Drawing for the job (mm, zero at the part's lowest x, y, z). A direction names the side the tool comes from. Round coordinates to 2 decimals unless told otherwise and drop trailing zeros. Write each loop counter-clockwise with the first axis right and the second up, starting at its lowest first coordinate (ties: lowest second). Pieces come first, ordered by that corner, then holes. Notation, with made-up numbers: (-25.75, -12.5) - (8.25, -12.5) arc R22 cw to (8.25, 26.5) - close; hole circle Ø9 at (14.25, -28). An arc over 180 degrees is marked (long way). Answer in a Markdown table with one row per item.
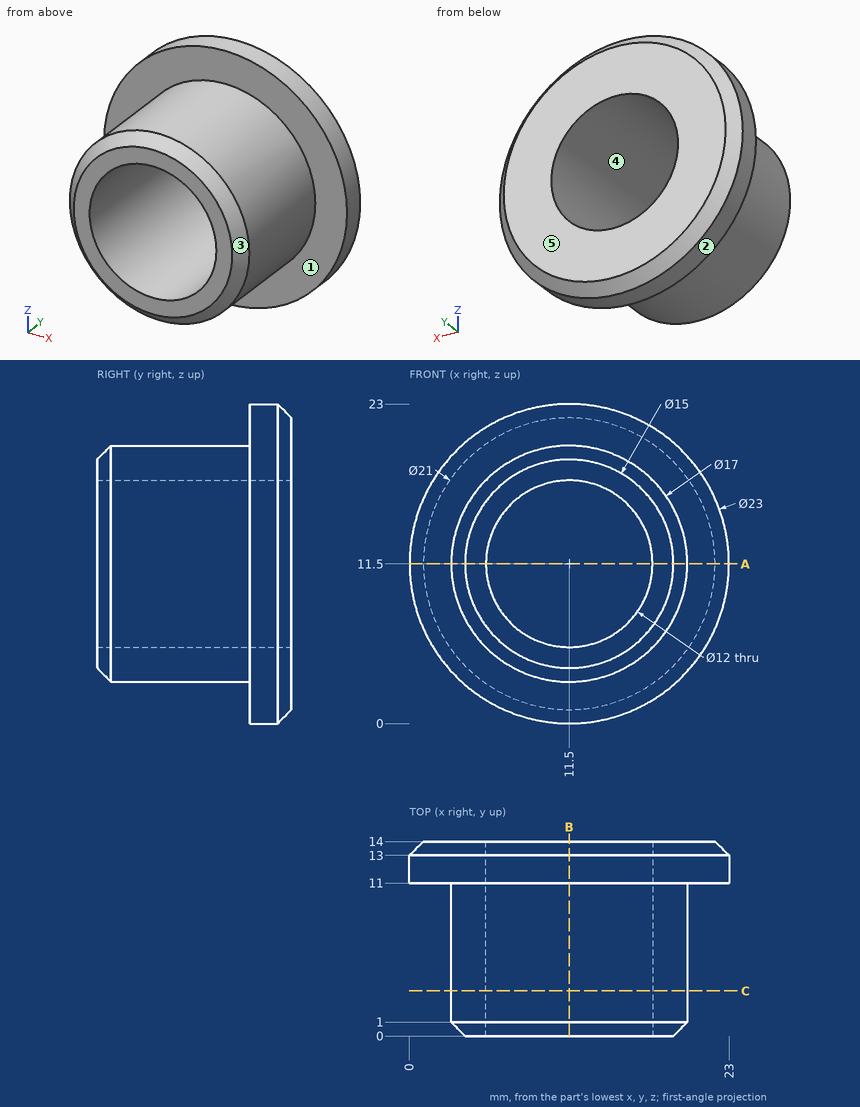
Q1. Saw through at B-B on x = 11.5. List the corners of the cut face in (y, z), then the cut area to 3 significant figures.
Computed:
| item | result |
|---|---|
| outline | (0, 4) - (1, 3) - (11, 3) - (11, 0) - (13, 0) - (14, 1) - (14, 5.5) - (0, 5.5) - close; (0, 17.5) - (14, 17.5) - (14, 22) - (13, 23) - (11, 23) - (11, 20) - (1, 20) - (0, 19) - close |
| area | 86.0 mm2 |
Q2. 3-axis set-ups, long thin cutter, end or side, ignore diameter. For the marked faces 1 and 2: which of +Z, -Z, +X, -X, +Y, -Y reach the whole face in a straight line?
Computed:
| item | result |
|---|---|
| face 1 | -Y |
| face 2 | +Y, -Y |
Q3. Saw through at A-A on z = 11.5. List the corners of the cut face in (x, y).
Computed:
| item | result |
|---|---|
| outline | (0, 11) - (3, 11) - (3, 1) - (4, 0) - (5.5, 0) - (5.5, 14) - (1, 14) - (0, 13) - close; (17.5, 0) - (19, 0) - (20, 1) - (20, 11) - (23, 11) - (23, 13) - (22, 14) - (17.5, 14) - close |
Q4. Pull direction Z, two halves, no side cores. Call the marked faces 3, 4 and 5: released by +Z, released by -Z, zero draft, split by the parting line, or undercut.
Computed:
| item | result |
|---|---|
| face 3 | split by the parting line |
| face 4 | undercut |
| face 5 | zero draft |
Q5. Saw through at C-C on y = 3.25. List the corners of the cut face in (x, z).
Computed:
| item | result |
|---|---|
| outline | circle Ø17 at (11.5, 11.5); hole circle Ø12 at (11.5, 11.5) |
Q6. Flat gauge pins, fed straight in: pin 1 (8 mm diameter, centred on y = 2.5, z = 10.5, fed in from -X); pin 2 (2 mm diameter, centred on y = 11, z = 14.5, fed in from -X); pin 3 (2 mm diameter, centred on x = 10.5, y = 7, fed in from +Z). Where does each tip first touch, or does it go through?
Computed:
| item | result |
|---|---|
| pin 1 | stops at x = 3 |
| pin 2 | stops at x = 0.18 |
| pin 3 | stops at z = 20 |
Q7. Drill centre lines: line 1 (Z direction, x = 11.5, y = 5.5); line 2 (Y direction, x = 20.75, z = 13.25); line 3 (X direction, y = 11.75, z = 9.25). Where is each one in solid material? Low to high.
Computed:
| item | result |
|---|---|
| line 1 | z = 3 to 5.5, 17.5 to 20 |
| line 2 | y = 11 to 14 |
| line 3 | x = 0.22 to 5.94, 17.06 to 22.78 |
